Read the model definition and answer for the solid it produces. Units are mm, in the model's axes. Face numbers are marked on the shaded views. A direction names the side the tool comes from. Coordinates: 2 decimals unless noted, no trailing zeros. Write each loop counter-clockwise with the first axis right and the second up, starting at its lowest first coordinate (ties: lowest second). Pieces come first, ordered by that corner, then holes.
Item 1: Straight lines are drawn through the part: probe 1 along X at (y, z) = (-18.5, -4) (3 decimals); probe 2 along Z at (x, y) = (38, 42.5) (3 decimals); probe 3 along Y at (x, z) = (20, 38.5) (3 decimals). For each, find the intervals that lie inside material, in ascending order.
Item 2: A tool of negligible diameter and unlimited length cuts with its end or side. For the marked faces 1, 2, 3 and 4, from which of +Z, -Z, +X, -X, +Y, -Y can it reach the whole face along a straight path? Write none if from no direction.
Item 3: Section B-B (y = 51) is taken. Give the vertices of the cut face in (x, z) (3 decimals).
Item 4: Section A-A (z = 5.5) is taken. Give the vertices of the cut face in (x, y) (3 decimals).
Item 5: Each of these flat-tipped pins is pushed along its axis until it touches: P1, Ø17, axis at x = 53.5, z = 36.5, coming from the -Y side; P2, Ø15.5, axis at x = 28, z = 34.5, coming from the +Y side; P3, Ø3, axis at x = 7.5, y = -50, coming from the +Z side (3 decimals); P4, Ø12, axis at y = -35, z = 54.5, coming from the +X side. Where does it stop, or does it pass through?
from build123d import *

# Parameters (mm, degrees)
F1_DEPTH = 63.5
F0_W     = 25.4
F0_H     = 19.05
F0_H_2   = 4.7498
F0_H_3   = 4.7752
F2_DEPTH = 25.4
F3_DEPTH = 3.175


with BuildPart() as f1:
    # F0 (on Front) → F1 (new body, symmetric)
    with BuildSketch(Plane.XZ):
        Polygon((-41.275, -9.525), (41.275, -9.525), (41.275, 9.525), (22.225, 9.525), (-41.275, 9.525), align=None)
    extrude(amount=F1_DEPTH, both=True)

    # F0 (on Front) → F2 (join, symmetric)
    with BuildSketch(Plane.XZ):
        with BuildLine():
            Line((22.225, 9.525), (41.275, 9.525))
            Line((41.275, 9.525), (41.275, 27.0002))
            ThreePointArc((41.275, 27.0002), (45.9246798487, 38.2255201513), (57.15, 42.8752))
            Line((57.15, 42.8752), (60.325, 42.8752))
            Line((60.325, 42.8752), (60.325, 61.9252))
            Line((60.325, 61.9252), (57.15, 61.9252))
            add(Edge.make_bspline(
                [(52.3907166691, 61.5994029847), (53.9548508267, 61.7140325614), (55.5412148436, 61.8226215769), (57.15, 61.9252)],
                knots=[109.0083952872, 109.0083952872, 109.0083952872, 109.0083952872, 111.5045361635, 111.5045361635, 111.5045361635, 111.5045361635], degree=3))
            ThreePointArc((52.3907166691, 61.5994029847), (30.8253575966, 49.9516449945), (22.225, 27.0002))
            Line((22.225, 27.0002), (22.225, 9.525))
        make_face()
        with Locations((73.025, 52.4002)):
            Rectangle(F0_W, F0_H)
        with Locations((73.025, 64.3001)):
            Rectangle(F0_W, F0_H_2)
        with Locations((73.025, 40.4876)):
            Rectangle(F0_W, F0_H_3)
    extrude(amount=F2_DEPTH, both=True)

    # F0 (on Front) → F3 (join, symmetric)
    with BuildSketch(Plane.XZ):
        with BuildLine():
            add(Edge.make_bspline(
                [(-41.275, 9.525), (-41.8278017588, 40.0673060795), (-15.9162271246, 56.5934410498), (52.3907166691, 61.5994029847)],
                knots=[0, 0, 0, 0, 109.0083952872, 109.0083952872, 109.0083952872, 109.0083952872], degree=3))
            Line((-41.275, 9.525), (22.225, 9.525))
            Line((22.225, 9.525), (22.225, 27.0002))
            ThreePointArc((22.225, 27.0002), (30.8253575966, 49.9516449945), (52.3907166691, 61.5994029847))
        make_face()
    extrude(amount=F3_DEPTH, both=True)

    # F0 (on Front) → F4 (revolve)
    with BuildSketch(Plane.XZ):
        Polygon((85.725, 61.9252), (85.725, 42.8752), (85.725, 38.1), (111.125, 38.1), (111.125, 66.675), (85.725, 66.675), align=None)
    revolve(axis=Axis((85.725, 0, 52.3875), (0, 0, 1)))


solid = f1.part
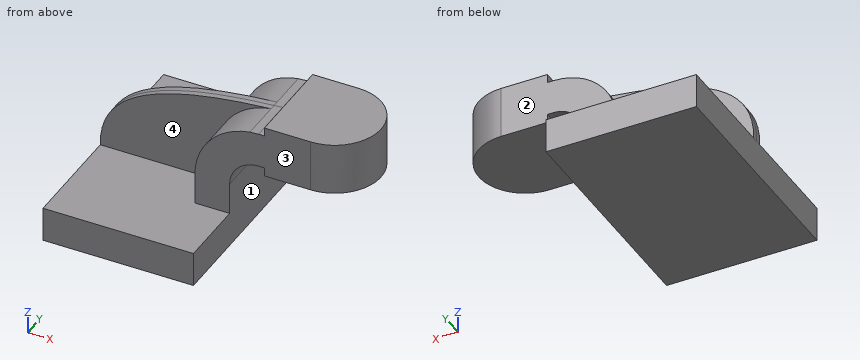
Established:
1. probe 1: x = -41.275 to 41.275
1. probe 2: z = -9.525 to 9.525
1. probe 3: y = -3.175 to 3.175
2. face 1: -Z, +X, +Y, -Y
2. face 2: +Z, +X, -X, +Y
2. face 3: +Z, +X, -X, -Y
2. face 4: +Z, -X, -Y
3. outline: (-41.275, -9.525) - (41.275, -9.525) - (41.275, 9.525) - (-41.275, 9.525) - close
4. outline: (-41.275, -63.5) - (41.275, -63.5) - (41.275, 63.5) - (-41.275, 63.5) - close
5. P1: stops at y = -25.4
5. P2: stops at y = 25.4
5. P3: stops at z = 9.525
5. P4: passes through
